Source: CAD feature listing. Evaluate the final solid. Frame: model axes, mm. A direction names the side the tool comes from. Round coordinates to 2 decimals unless told otherwise and drop trailing zeros. Loops run counter-clockwise (first coordinate to the right, second up) from the corner with the lowest first, then second, coordinate; pieces in that order, holes last.
Item 1: First-contact query: P1, Ø10, axis at x = 5.5, z = 1, coming from the +Y side; P2, Ø1, axis at x = -8, z = -3.5, coming from the -Y side. Flat tips, straight axial feed; report the tip coordinate or a pass-through.
Item 2: Section query A-A on y = -5.5. Return loops of the section in (x, z), then the cut area to 3 significant figures.
Item 3: Access query for faces 4 (the flat face through (13.52, -37.14, 0.18)), 5 (the flat face through (11.112, 40, 0)), 6 (the flat face through (-11.112, -40, 0)). Directions: +Z, -Z, +X, -X, +Y, -Y. A direction counts if a zero-diameter tool reaches every point of the face in a straight line with its end or side. Return the directions, or none.
Item 4: Ray query, L1, parallel to X at y = 4, z = -7.25; L2, parallel to Y at x = 13.5, z = 9.25 (3 decimals); L3, parallel to Y at x = 3, z = 11.75. Return the intervals inside material, ascending.
Item 5: Section query C-C on x = 6.5. Return loops of the section in (y, z), then the cut area to 3 significant figures.
Item 6: Pull-direction query (Y, two-part tool) for faces 1 (the flat face through (0, 0, 12.7)), 2 (the flat face through (-15, -38.506, 0)), 3 (the flat face through (-16, -41.275, 0)); classes: released by +Y, released by -Y, zero draft, split by the parting line, or undercut.
Item 7: Section query B-B on x = -15.5. Return loops of the section in (y, z) (3 decimals).
```python
from build123d import *

# Parameters (mm, degrees)
BASE_EXTRUDE_DEPTH = 12.7


with BuildPart() as part:
    # Sketch1 → Base-Extrude (new, symmetric)
    with BuildSketch(Plane.XY):
        with BuildLine():
            Line((-11.1125, 41.275), (-20.6375, 41.275))
            Line((-20.6375, 41.275), (-20.6375, -41.275))
            Line((-20.6375, -41.275), (-11.1125, -41.275))
            Line((-11.1125, -41.275), (-11.1125, -38.5064))
            Line((-11.1125, -38.5064), (-12.710951958, -35.7378))
            Line((-12.710951958, -35.7378), (-14.309403911, -38.5064))
            Line((-14.309403911, -38.5064), (-16.4846, -38.5064))
            ThreePointArc((-16.4846, -38.5064), (-17.463447917, -38.100947917), (-17.8689, -37.1221))
            Line((-17.8689, -37.1221), (-17.8689, -2.7686))
            ThreePointArc((-17.8689, -2.7686), (-17.463447917, -1.789752083), (-16.4846, -1.3843))
            Line((-16.4846, -1.3843), (16.4846, -1.3843))
            ThreePointArc((16.4846, -1.3843), (17.463447917, -1.789752083), (17.8689, -2.7686))
            Line((17.8689, -2.7686), (17.8689, -37.1221))
            ThreePointArc((17.8689, -37.1221), (17.463447917, -38.100947917), (16.4846, -38.5064))
            Line((16.4846, -38.5064), (14.309403911, -38.5064))
            Line((14.309403911, -38.5064), (12.710951958, -35.7378))
            Line((12.710951958, -35.7378), (11.1125, -38.5064))
            Line((11.1125, -38.5064), (11.1125, -41.275))
            Line((11.1125, -41.275), (20.6375, -41.275))
            Line((20.6375, -41.275), (20.6375, 41.275))
            Line((20.6375, 41.275), (11.1125, 41.275))
            Line((11.1125, 41.275), (11.1125, 38.5064))
            Line((11.1125, 38.5064), (12.710951958, 35.7378))
            Line((12.710951958, 35.7378), (14.309403911, 38.5064))
            Line((14.309403911, 38.5064), (16.4846, 38.5064))
            ThreePointArc((16.4846, 38.5064), (17.463447917, 38.100947917), (17.8689, 37.1221))
            Line((17.8689, 37.1221), (17.8689, 2.7686))
            ThreePointArc((17.8689, 2.7686), (17.463447917, 1.789752083), (16.4846, 1.3843))
            Line((16.4846, 1.3843), (-16.4846, 1.3843))
            ThreePointArc((-16.4846, 1.3843), (-17.463447917, 1.789752083), (-17.8689, 2.7686))
            Line((-17.8689, 2.7686), (-17.8689, 37.1221))
            ThreePointArc((-17.8689, 37.1221), (-17.463447917, 38.100947917), (-16.4846, 38.5064))
            Line((-16.4846, 38.5064), (-14.309403911, 38.5064))
            Line((-14.309403911, 38.5064), (-12.710951958, 35.7378))
            Line((-12.710951958, 35.7378), (-11.1125, 38.5064))
            Line((-11.1125, 38.5064), (-11.1125, 41.275))
        make_face()
    extrude(amount=BASE_EXTRUDE_DEPTH, both=True)


solid = part.part
```
Data:
1. P1: stops at y = 1.38
1. P2: stops at y = -1.38
2. outline: (-20.64, -12.7) - (-17.87, -12.7) - (-17.87, 12.7) - (-20.64, 12.7) - close; (17.87, -12.7) - (20.64, -12.7) - (20.64, 12.7) - (17.87, 12.7) - close
2. area: 141 mm2
3. face 4: +Z, -Z
3. face 5: +Z, -Z, +Y
3. face 6: +Z, -Z, -Y
4. L1: x = -20.64 to -17.87, 17.87 to 20.64
4. L2: y = -41.275 to -37.104, -1.384 to 1.384, 37.104 to 41.275
4. L3: y = -1.38 to 1.38
5. outline: (-1.38, -12.7) - (1.38, -12.7) - (1.38, 12.7) - (-1.38, 12.7) - close
5. area: 70.3 mm2
6. face 1: zero draft
6. face 2: undercut
6. face 3: released by -Y
7. outline: (-41.275, -12.7) - (-38.506, -12.7) - (-38.506, 12.7) - (-41.275, 12.7) - close; (-1.384, -12.7) - (1.384, -12.7) - (1.384, 12.7) - (-1.384, 12.7) - close; (38.506, -12.7) - (41.275, -12.7) - (41.275, 12.7) - (38.506, 12.7) - close
